```python
from build123d import *

# Parameters (mm, degrees)
SKETCH1_W                         = 254
SKETCH1_H                         = 114.3
BOSS_EXTRUDE1_DEPTH               = 6.35
SKETCH2_R                         = 11
CUT_EXTRUDE1_DEPTH                = 140.411064841
F_3_8_CLEARANCE_HOLE1_D           = 10.31748
F_3_8_CLEARANCE_HOLE1_CSINK_D     = 11.58748
F_3_8_CLEARANCE_HOLE1_CSINK_ANGLE = 90


with BuildPart() as part:
    # Sketch1 → Boss-Extrude1 (new body)
    with BuildSketch(Plane(origin=(0, 0, 0), x_dir=(1, 0, 0), z_dir=(0, 1, 0))):
        Rectangle(SKETCH1_W, SKETCH1_H)
    extrude(amount=BOSS_EXTRUDE1_DEPTH)

    # Sketch2 → Cut-Extrude1 (cut, through all)
    with BuildSketch(Plane(origin=(0, 6.35, 0), x_dir=(1, 0, 0), z_dir=(0, 1, 0))):
        with Locations(Location((-107.475, 0, 0), (0, 0, 270))):
            Circle(SKETCH2_R)
    extrude(amount=-CUT_EXTRUDE1_DEPTH, mode=Mode.SUBTRACT)

    # 3/8 Clearance Hole1 (through all)
    with Locations(Plane(origin=(0, 6.35, 0), x_dir=(1, 0, 0), z_dir=(0, 1, 0))):
        with Locations((112.7125, 42.8625), (112.7125, -42.8675), (-112.7175, -42.8675), (-112.7175, 42.8625)):
            CounterSinkHole(F_3_8_CLEARANCE_HOLE1_D / 2, F_3_8_CLEARANCE_HOLE1_CSINK_D / 2, counter_sink_angle=F_3_8_CLEARANCE_HOLE1_CSINK_ANGLE)


solid = part.part
```
Part model, mm, in its own coordinate system. Round coordinates to 2 decimals unless told otherwise and drop trailing zeros. Loops run counter-clockwise (first coordinate to the right, second up) from the corner with the lowest first, then second, coordinate; pieces in that order, holes last. Notation, with made-up numbers: (43.25, 78) -> (77.25, 78) arc R16 cw to (77.25, 88) -> close; hole circle Ø3 at (26.5, -39.5). An arc over 180 degrees is marked (long way). Use CSV: the item, a comma, the result in double quotes. Start each with the question number.
1) Wall check: L1, parallel to Z at x = 112, y = 3.75; L2, parallel to X at y = 2, z = 1; L3, parallel to X at y = 5.5, z = -45.5. Give the ranges that are in metal, low to high. Write a range as [from, to].
2) Cut at B-B, the plane y = 2. Give the number of separate pieces and of enclosed holes in the cut face, plus the area to 3 significant figures.
3) Pull direction X, two halves, no side cores. Call faces 1 (the flat face through (127, 3, 1)), 2 (the cylindrical face through (-108.624, 2.817, 46.007)), 3 (the flat face through (-2, 3, 57.15)): +X half, -X half, draft (parallel to the pull), parting line (faces both ways), or undercut.
4) Cut at A-A, the plane z = 0. Write the cut outline in (x, y) (3 decimals).
5) Drop a flat-ended pin along its axis: P1, Ø1, axis at x = -92, z = -30.5, coming from the -Y side. Give the stop position or say it passes through.
Determined:
1,L1,"z = [-57.15, -47.97], [-37.75, 37.76], [47.98, 57.15]"
1,L2,"x = [-127, -118.43], [-96.52, 127]"
1,L3,"x = [-127, -117.15], [-108.28, 108.28], [117.15, 127]"
2,separate pieces,"1"
2,enclosed holes,"5"
2,area,"28,300 mm2"
3,face 1,"+X half"
3,face 2,"undercut"
3,face 3,"draft"
4,outline,"(-127, 0) -> (-118.475, 0) -> (-118.475, 6.35) -> (-127, 6.35) -> close; (-96.475, 0) -> (127, 0) -> (127, 6.35) -> (-96.475, 6.35) -> close"
5,P1,"stops at y = 0"
